Verification items for the finished model (mm, model axes). A direction names the side the tool comes from. Round coordinates to 2 decimals unless told otherwise and drop trailing zeros. Loops run counter-clockwise (first coordinate to the right, second up) from the corner with the lowest first, then second, coordinate; pieces in that order, holes last. Notation, with made-up numbers: (51, 85) - (89, 85) arc R15 ccw to (89, 91) - close; hole circle Ø4 at (64.5, 63.5). An arc over 180 degrees is marked (long way). Use a Markdown table: item, result. Add a question column.
```python
from build123d import *

# Parameters (mm, degrees)
SKETCH_1_W           = 80
SKETCH_1_H           = 150
EXTRUDE_1_DEPTH      = 10
SKETCH_4_R           = 11.25
EXTRUDE_3_DEPTH      = 10
SKETCH_5_R           = 11.25
SKETCH_5_R_2         = 5
EXTRUDE_4_DEPTH      = 4
SKETCH_6_R           = 2.1
CUT_EXTRUDE_1_DEPTH  = 24
SKETCH_7_W           = 3.4
SKETCH_7_H           = 7.5
CUT_EXTRUDE_2_DEPTH  = 24
SKETCH_8_R           = 2.1
CUT_EXTRUDE_3_DEPTH  = 24
SKETCH_9_W           = 80
SKETCH_9_H           = 40
SKETCH_9_R           = 11
SKETCH_9_R_2         = 1.6
EXTRUDE_5_DEPTH      = 10
FILLET_1_R           = 5
SKETCH_10_W          = 3.4
SKETCH_10_H          = 7.5
CUT_EXTRUDE_5_DEPTH  = 10
SKETCH_11_R          = 2.1
CUT_EXTRUDE_6_DEPTH  = 24
SKETCH_12_R          = 2.1
CUT_EXTRUDE_7_DEPTH  = 24
SKETCH_14_W          = 4
SKETCH_14_H          = 2
CUT_EXTRUDE_9_DEPTH  = 10
SKETCH_16_R          = 2.1
CUT_EXTRUDE_10_DEPTH = 11


with BuildPart() as part:
    # 草圖1 → 填料-伸長1 (new body)
    with BuildSketch(Plane.XY):
        Rectangle(SKETCH_1_W, SKETCH_1_H)
    extrude(amount=EXTRUDE_1_DEPTH)

    # 草圖4 → 填料-伸長3 (add)
    with BuildSketch(Plane.XZ.offset(75)):
        with BuildLine():
            ThreePointArc((-6, 49), (0, 43), (6, 49))
            Line((6, 49), (6, 50))
            Line((6, 50), (29, 50))
            Line((29, 50), (29, 27.881405907))
            ThreePointArc((29, 27.881405907), (30, 21.95), (31, 27.881405907))
            Line((31, 27.881405907), (31, 50))
            Line((31, 50), (40, 50))
            Line((40, 50), (40, 10))
            Line((40, 10), (-40, 10))
            Line((-40, 10), (-40, 50))
            Line((-40, 50), (-31, 50))
            Line((-31, 50), (-31, 27.881405907))
            ThreePointArc((-31, 27.881405907), (-30, 21.95), (-29, 27.881405907))
            Line((-29, 27.881405907), (-29, 50))
            Line((-29, 50), (-6, 50))
            Line((-6, 50), (-6, 49))
        make_face()
        with Locations((0, 25)):
            Circle(SKETCH_4_R, mode=Mode.SUBTRACT)
    extrude(amount=-EXTRUDE_3_DEPTH)

    # 草圖5 → 填料-伸長4 (add)
    with BuildSketch(Plane.XZ.offset(75)):
        with Locations((0, 25)):
            Circle(SKETCH_5_R)
        with Locations((0, 25)):
            Circle(SKETCH_5_R_2, mode=Mode.SUBTRACT)
    extrude(amount=-EXTRUDE_4_DEPTH)

    # 草圖6 → 除料-伸長1 (cut)
    with BuildSketch(Plane(origin=(40, 0, 0), x_dir=(0, 0, -1), z_dir=(1, 0, 0))):
        with Locations((-40, -70)):
            Circle(SKETCH_6_R)
    extrude(amount=-CUT_EXTRUDE_1_DEPTH, mode=Mode.SUBTRACT)

    # 草圖7 → 除料-伸長2 (cut)
    with BuildSketch(Plane.XZ.offset(75)):
        with Locations((-21.943112787, 40)):
            Rectangle(SKETCH_7_W, SKETCH_7_H)
        with Locations((21.943112787, 40)):
            Rectangle(SKETCH_7_W, SKETCH_7_H)
    extrude(amount=-CUT_EXTRUDE_2_DEPTH, mode=Mode.SUBTRACT)

    # 草圖8 → 除料-伸長3 (cut)
    with BuildSketch(Plane.ZY.offset(40)):
        with Locations((40, -70)):
            Circle(SKETCH_8_R)
    extrude(amount=-CUT_EXTRUDE_3_DEPTH, mode=Mode.SUBTRACT)

    # 草圖9 → 填料-伸長5 (add)
    with BuildSketch(Plane(origin=(0, 75, 0), x_dir=(1, 0, 0), z_dir=(0, 1, 0))):
        with Locations((0, -30)):
            Rectangle(SKETCH_9_W, SKETCH_9_H)
        with Locations((0, -25)):
            Circle(SKETCH_9_R, mode=Mode.SUBTRACT)
        with Locations((-21.920310217, -25)):
            Circle(SKETCH_9_R_2, mode=Mode.SUBTRACT)
        with Locations((0, -46.920310217)):
            Circle(SKETCH_9_R_2, mode=Mode.SUBTRACT)
        with Locations((21.920310217, -25)):
            Circle(SKETCH_9_R_2, mode=Mode.SUBTRACT)
    extrude(amount=-EXTRUDE_5_DEPTH)

    # 圓角1
    fillet_1_edges = [part.edges().sort_by_distance(p)[0] for p in [
        (40, 70, 50),
        (-40, 70, 50),
        (40, -70, 50),
        (-40, -70, 50),
    ]]
    fillet(fillet_1_edges, radius=FILLET_1_R)

    # 草圖10 → 除料-伸長5 (cut)
    with BuildSketch(Plane(origin=(0, 75, 0), x_dir=(1, 0, 0), z_dir=(0, 1, 0))):
        with BuildLine():
            Line((-30.992105359, -72.117230176), (-29, -72.117230176))
            Line((-29, -72.117230176), (-29, -27.881405907))
            ThreePointArc((-29, -27.881405907), (-30.004176302, -21.950002859), (-30.992105359, -27.884133658))
            Line((-30.992105359, -27.884133658), (-30.992105359, -72.117230176))
        make_face()
        with BuildLine():
            Line((29.001577897, -72.118320527), (31, -72.118320527))
            Line((31, -72.118320527), (31, -27.881405907))
            ThreePointArc((31, -27.881405907), (29.999164969, -21.950000114), (29.001577897, -27.881953036))
            Line((29.001577897, -27.881953036), (29.001577897, -72.118320527))
        make_face()
        with Locations((-21.943112787, -40)):
            Rectangle(SKETCH_10_W, SKETCH_10_H)
        with Locations((21.943112787, -40)):
            Rectangle(SKETCH_10_W, SKETCH_10_H)
    extrude(amount=-CUT_EXTRUDE_5_DEPTH, mode=Mode.SUBTRACT)

    # 草圖11 → 除料-伸長6 (cut)
    with BuildSketch(Plane(origin=(40, 0, 0), x_dir=(0, 0, -1), z_dir=(1, 0, 0))):
        with Locations((-40, 70)):
            Circle(SKETCH_11_R)
    extrude(amount=-CUT_EXTRUDE_6_DEPTH, mode=Mode.SUBTRACT)

    # 草圖12 → 除料-伸長7 (cut)
    with BuildSketch(Plane.ZY.offset(40)):
        with Locations((40, 70)):
            Circle(SKETCH_12_R)
    extrude(amount=-CUT_EXTRUDE_7_DEPTH, mode=Mode.SUBTRACT)

    # 草圖14 → 除料-伸長9 (cut)
    with BuildSketch(Plane.XZ.offset(75)):
        with Locations((-12, 46)):
            Rectangle(SKETCH_14_W, SKETCH_14_H)
        with Locations((12, 46)):
            Rectangle(SKETCH_14_W, SKETCH_14_H)
    extrude(amount=-CUT_EXTRUDE_9_DEPTH, mode=Mode.SUBTRACT)

    # 草圖16 → 除料-伸長10 (cut, through all)
    with BuildSketch(Plane.XY.offset(10)):
        with Locations((-20, 37.5)):
            Circle(SKETCH_16_R)
        with Locations((20, 37.5)):
            Circle(SKETCH_16_R)
        with Locations((20, -37.5)):
            Circle(SKETCH_16_R)
        with Locations((-20, -37.5)):
            Circle(SKETCH_16_R)
    extrude(amount=-CUT_EXTRUDE_10_DEPTH, mode=Mode.SUBTRACT)


solid = part.part
```
Q1. Go/stop test with flat-tipped pins: pin 1 Ø1.1 at (y, z) = (-69.5, 49.5) entering from +X; pin 2 Ø5 at (x, y) = (-8.5, -57) entering from +Z; pin 3 Ø0.6 at (y, z) = (-71.5, 45.5) entering from +X. Record where each tip stops, or that it passes through.
Q2. Thickness scan on line 1 along X through (y, z) = (71.25, 25); line 2 along Y through (x, z) = (-19, 15.5); line 3 along Y through (x, z) = (-20, 41.5). Record the ranges inside material, lowest first.
Q3. Set-up check for faces 1 (the face through (31, 72.3, 39.1)), 2 (the face through (-22, -70, 36.25)), 3 (the face through (-18.151, 68.722, 38.334)): record each of +Z, -Z, +X, -X, +Y, -Y from which the full face is reachable in a straight line by a thin tool's end or side.
Q4. Section check A-A on y = 37.5. Record the cut outline in (x, z), plus the area to 3 significant figures.
Q5. Release check for a two-part mould opening along X. For faces 4 (the face through (0.74, 70.07, 48.34)), 5 (the face through (33, 70, 50)), 6 (the face through (-16, -70, 40)), 7 (the face through (22, -70, 43.75)) record: +X half, -X half, draft (parallel to the pull), parting line (faces both ways), or undercut.
Determined:
| question | item | result |
|---|---|---|
| 1 | pin 1 | stops at x = 38.07 |
| 1 | pin 2 | stops at z = 10 |
| 1 | pin 3 | stops at x = 40 |
| 2 | line 1 | x = -40 to -33.05, -26.95 to -23.52, -20.32 to -11, 11 to 20.32, 23.52 to 26.95, 33.05 to 40 |
| 2 | line 2 | y = -75 to -65, 65 to 75 |
| 2 | line 3 | y = -75 to -71.47, -68.53 to -65, 65 to 68.53, 71.47 to 75 |
| 3 | face 1 | +Z, +Y, -Y |
| 3 | face 2 | +Y, -Y |
| 3 | face 3 | -X |
| 4 | outline | (-40, 0) - (-22.1, 0) - (-22.1, 10) - (-40, 10) - close; (-17.9, 0) - (17.9, 0) - (17.9, 10) - (-17.9, 10) - close; (22.1, 0) - (40, 0) - (40, 10) - (22.1, 10) - close |
| 4 | area | 716 mm² |
| 5 | face 4 | undercut |
| 5 | face 5 | draft |
| 5 | face 6 | -X half |
| 5 | face 7 | undercut |
